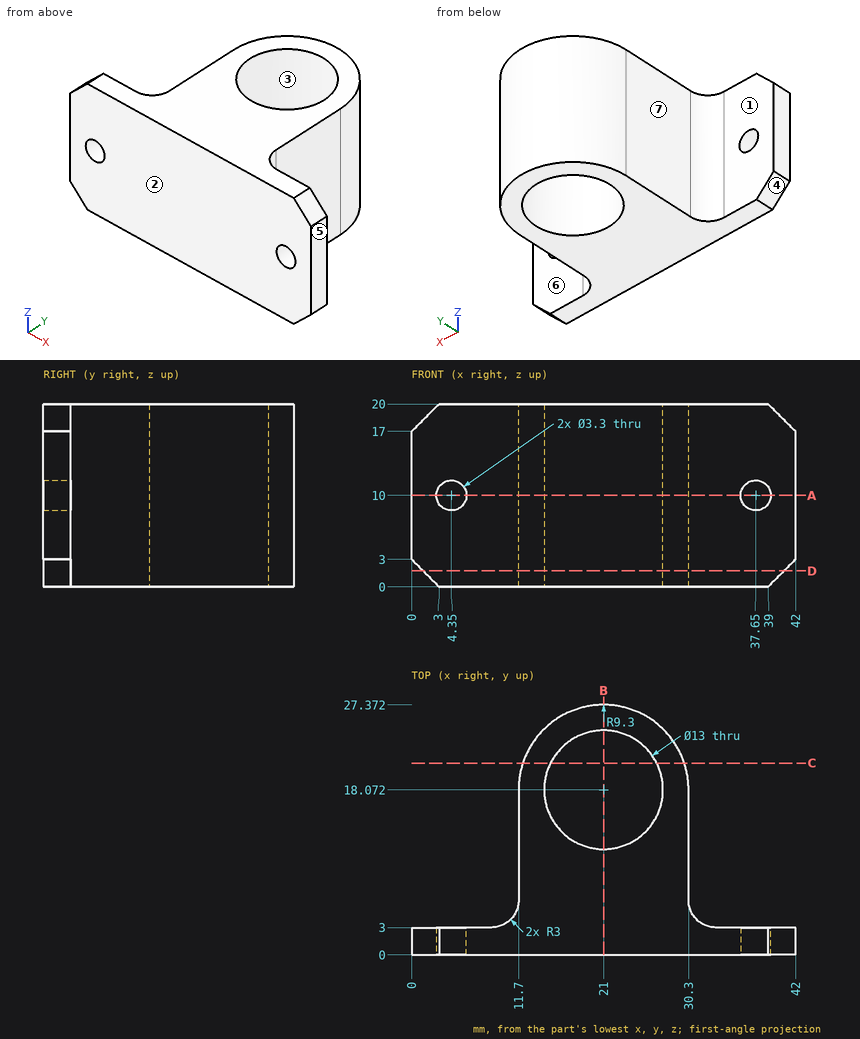
Here's the drawing with two shaded views (mm, measured from the low corner). I have some questions. A direction names the side the tool comes from. Round coordinates to 2 decimals unless told otherwise and drop trailing zeros. Loops run counter-clockwise (first coordinate to the right, second up) from the corner with the lowest first, then second, coordinate; pieces in that order, holes last. Notation, with made-up numbers: (-26, 11) -> (24, 11) arc R22 ccw to (24, 35) -> close; hole circle Ø9 at (67, 13). An arc over 180 degrees is marked (long way). Answer as CSV lines item,"result". Start each with the question number.
1. If we mould it in two halves opening along Y, with no side actions, what happens to the marked faces 1, 2, 3 and 4? For each: pulls with the +Y half, pulls with the -Y half, needs draft (parallel to the pull), parting line crosses it, or undercut.
2. For the marked faces 5, 6 and 7, which set-ups out of +Z, -Z, +X, -X, +Y, -Y let a thin tool reach every point of the face, with its end or its side?
3. Imagine slicing it at B-B on x = 21. Write out the boundary of the cut face in (y, z).
4. Imagine slicing it at A-A on z = 10. Write out the boundary of the cut face in (x, y).
5. Imagine slicing it at C-C on y = 21. Write out the boundary of the cut face in (x, z), plus the area to 3 significant figures.
6. I need wall thicknesses on probe 1 along Z at (x, y) = (37.65, 2); probe 2 along Y at (x, z) = (2, 12.5); probe 3 along X at (y, z) = (21.5, 6.75) (1 decimal). Which ranges of each line are inside material? Lowest first, please. Write a range as from..to.
7. I'm going to push flat-ended pins straight in: P1, Ø2, axis at y = 10.5, z = 16, coming from the +X side; P2, Ø2.5, axis at x = 39, z = 12, coming from the +Y side; P3, Ø4, axis at y = 24, z = 11, coming from the +X side. Where does each tip first touch, or does it pass through?
8. Imagine slicing it at D-D on z = 1.75. Write out the boundary of the cut face in (x, y).
Solution:
1,face 1,"pulls with the +Y half"
1,face 2,"pulls with the -Y half"
1,face 3,"undercut"
1,face 4,"needs draft"
2,face 5,"+Z, -Z, +X, +Y, -Y"
2,face 6,"+Z, -Z, +X, +Y"
2,face 7,"+Z, -Z, -X, +Y"
3,outline,"(0, 0) -> (11.57, 0) -> (11.57, 20) -> (0, 20) -> close; (24.57, 0) -> (27.37, 0) -> (27.37, 20) -> (24.57, 20) -> close"
4,outline,"(0, 0) -> (2.7, 0) -> (2.7, 3) -> (0, 3) -> close; (6, 0) -> (36, 0) -> (36, 3) -> (33.3, 3) arc R3 cw to (30.3, 6) -> (30.3, 18.07) arc R9.3 ccw to (11.7, 18.07) -> (11.7, 6) arc R3 cw to (8.7, 3) -> (6, 3) -> close; (39.3, 0) -> (42, 0) -> (42, 3) -> (39.3, 3) -> close; hole circle Ø13 at (21, 18.07)"
5,outline,"(12.17, 0) -> (15.2, 0) -> (15.2, 20) -> (12.17, 20) -> close; (26.8, 0) -> (29.83, 0) -> (29.83, 20) -> (26.8, 20) -> close"
5,area,"121 mm²"
6,probe 1,"0..8.35, 11.65..20"
6,probe 2,"0..3"
6,probe 3,"12.4..15.5, 26.5..29.6"
7,P1,"x = 30.3"
7,P2,"y = 3"
7,P3,"x = 29.43"
8,outline,"(1.25, 0) -> (40.75, 0) -> (40.75, 3) -> (33.3, 3) arc R3 cw to (30.3, 6) -> (30.3, 18.07) arc R9.3 ccw to (11.7, 18.07) -> (11.7, 6) arc R3 cw to (8.7, 3) -> (1.25, 3) -> close; hole circle Ø13 at (21, 18.07)"
